Source: CAD feature listing. Evaluate the final solid. Frame: model axes, mm. Face numbers are marked on the shaded views. A direction names the side the tool comes from. Coordinates: 2 decimals unless noted, no trailing zeros. Order: outer loops, then holes, each group sorted by start corner. A loop starts at its lowest first (then second) coordinate and runs counter-clockwise, first axis right, second up. Notation, with made-up numbers: (21, 27) - (39, 27) arc R14 ccw to (39, 41) - close; hole circle Ø4 at (78, -23.5). An arc over 180 degrees is marked (long way). One line per question, with ' | ' between items. Start each with the question number.
(1) Contact query for flat-ended pins moving along their axis: P1, Ø1, axis at x = -7, y = 3, coming from the -Z side; P2, Ø0.6, axis at x = 0, z = 2, coming from the +Y side; P3, Ø1.6, axis at y = -9, z = 1.5, coming from the -X side. Output: stop coordinate, or through.
(2) Draft query along Y for the marked faces 1, 2 and 3. Return one class per face: +Y half, -Y half, draft (parallel to the pull), parting line (faces both ways), or undercut.
(3) Section B-B (x = 0). Return the cut outline in (y, z), then the cut area to 3 significant figures.
(4) Section A-A (z = 1.55). Return the cut outline in (x, y).
(5) Line query: line 1 along Y through (x, z) = (1.25, 1.35); line 2 along X through (y, z) = (5.75, 2); line 3 along X through (y, z) = (1.25, 2.65). Output: solid intervals per line, ascending.
(6) Access query for the marked faces 4, 5, 6 and 7. Directions: +Z, -Z, +X, -X, +Y, -Y. A direction counts if a zero-diameter tool reaches every point of the face in a straight line with its end or side. Return the directions, or none.
(7) Section D-D (y = 10). Return the cut outline in (x, z), then the cut area to 3 significant figures.
(8) Section C-C (y = 0). Return the cut outline in (x, z), then the cut area to 3 significant figures.
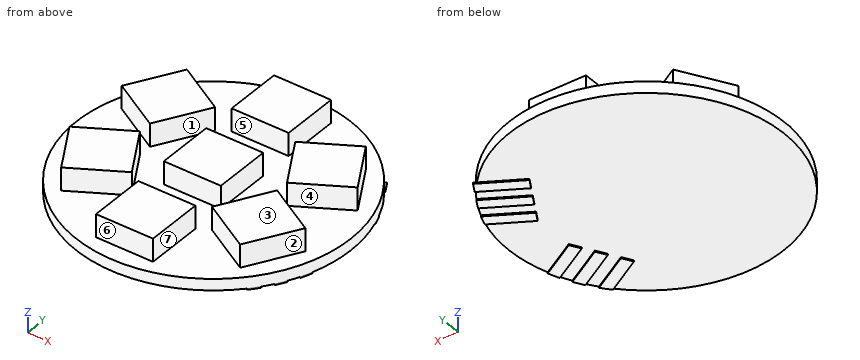
from build123d import *

# Parameters (mm, degrees)
CROQUIS1_R              = 12
SALIENTE_EXTRUIR1_DEPTH = 1
CROQUIS2_W              = 5
CROQUIS2_H              = 5
SALIENTE_EXTRUIR2_DEPTH = 2
SALIENTE_EXTRUIR3_DEPTH = 0.1


with BuildPart() as part:
    # Croquis1 → Saliente-Extruir1 (new body)
    with BuildSketch(Plane.XY):
        Circle(CROQUIS1_R)
    extrude(amount=SALIENTE_EXTRUIR1_DEPTH)

    # Croquis2 → Saliente-Extruir2 (add)
    with BuildSketch(Plane.XY.offset(1)):
        Rectangle(CROQUIS2_W, CROQUIS2_H)
        with Locations((0, -8)):
            Rectangle(CROQUIS2_W, CROQUIS2_H)
        with Locations((0, 8)):
            Rectangle(CROQUIS2_W, CROQUIS2_H)
        Polygon((-7.84326674, 7.415063509), (-10.34326674, 3.084936491), (-6.013139721, 0.584936491), (-3.513139721, 4.915063509), align=None)
        Polygon((-6.013139721, -0.584936491), (-10.34326674, -3.084936491), (-7.84326674, -7.415063509), (-3.513139721, -4.915063509), align=None)
        Polygon((6.013139721, -0.584936491), (3.513139721, -4.915063509), (7.84326674, -7.415063509), (10.34326674, -3.084936491), align=None)
        Polygon((7.84326674, 7.415063509), (3.513139721, 4.915063509), (6.013139721, 0.584936491), (10.34326674, 3.084936491), align=None)
    extrude(amount=SALIENTE_EXTRUIR2_DEPTH)

    # Croquis3 → Saliente-Extruir3 (add)
    with BuildSketch(Plane(origin=(0, 0, 0), x_dir=(-1, 0, 0), z_dir=(0, 0, -1))):
        with BuildLine():
            ThreePointArc((-9.560795314, -7.251978556), (-9.245794779, -7.649528018), (-8.914275675, -8.033410807))
            Line((-8.914275675, -8.033410807), (-5.67820323, -6.165063509))
            Line((-5.67820323, -6.165063509), (-6.17820323, -5.299038106))
            Line((-6.17820323, -5.299038106), (-9.560795314, -7.251978556))
        make_face()
        with BuildLine():
            Line((-7.17820323, -3.566987298), (-10.633279829, -5.561776702))
            ThreePointArc((-10.633279829, -5.561776702), (-10.515075861, -5.78214317), (-10.392305608, -5.999998679))
            ThreePointArc((-10.392305608, -5.999998679), (-10.265021594, -6.215249929), (-10.133279829, -6.427802106))
            Line((-10.133279829, -6.427802106), (-6.67820323, -4.433012702))
            Line((-6.67820323, -4.433012702), (-7.17820323, -3.566987298))
        make_face()
        with BuildLine():
            Line((-8.17820323, -1.834936491), (-11.414275675, -3.703283788))
            ThreePointArc((-11.414275675, -3.703283788), (-11.24758298, -4.182329148), (-11.060795314, -4.653902344))
            Line((-11.060795314, -4.653902344), (-7.67820323, -2.700961894))
            Line((-7.67820323, -2.700961894), (-8.17820323, -1.834936491))
        make_face()
        with BuildLine():
            Line((-7.67820323, 2.700961894), (-11.060795314, 4.653902344))
            ThreePointArc((-11.060795314, 4.653902344), (-11.24758298, 4.182329148), (-11.414275675, 3.703283788))
            Line((-11.414275675, 3.703283788), (-8.17820323, 1.834936491))
            Line((-8.17820323, 1.834936491), (-7.67820323, 2.700961894))
        make_face()
        with BuildLine():
            ThreePointArc((-10.133279829, 6.427802106), (-10.265021594, 6.215249929), (-10.392305608, 5.999998679))
            ThreePointArc((-10.392305608, 5.999998679), (-10.515075861, 5.78214317), (-10.633279829, 5.561776702))
            Line((-10.633279829, 5.561776702), (-7.17820323, 3.566987298))
            Line((-7.17820323, 3.566987298), (-6.67820323, 4.433012702))
            Line((-6.67820323, 4.433012702), (-10.133279829, 6.427802106))
        make_face()
        Polygon((-9.642304845, 7.299038106), (-6.17820323, 5.299038106), (-5.67820323, 6.165063509), (-9.142304845, 8.165063509), align=None)
    extrude(amount=SALIENTE_EXTRUIR3_DEPTH)


solid = part.part
Response values:
1) P1: stops at z = 0 | P2: stops at y = 10.5 | P3: stops at x = -8.59
2) face 1: undercut | face 2: -Y half | face 3: draft
3) outline: (-12, 0) - (12, 0) - (12, 1) - (10.5, 1) - (10.5, 3) - (5.5, 3) - (5.5, 1) - (2.5, 1) - (2.5, 3) - (-2.5, 3) - (-2.5, 1) - (-5.5, 1) - (-5.5, 3) - (-10.5, 3) - (-10.5, 1) - (-12, 1) - close | area: 54.0 mm²
4) outline: (-10.34, -3.08) - (-7.84, -7.42) - (-3.51, -4.92) - (-6.01, -0.58) - close; (-10.34, 3.08) - (-6.01, 0.58) - (-3.51, 4.92) - (-7.84, 7.42) - close; (-2.5, -10.5) - (2.5, -10.5) - (2.5, -5.5) - (-2.5, -5.5) - close; (-2.5, -2.5) - (2.5, -2.5) - (2.5, 2.5) - (-2.5, 2.5) - close; (-2.5, 5.5) - (2.5, 5.5) - (2.5, 10.5) - (-2.5, 10.5) - close; (3.51, -4.92) - (7.84, -7.42) - (10.34, -3.08) - (6.01, -0.58) - close; (3.51, 4.92) - (6.01, 0.58) - (10.34, 3.08) - (7.84, 7.42) - close
5) line 1: y = -10.5 to -5.5, -2.5 to 2.5, 5.5 to 10.5 | line 2: x = -8.8 to -4.96, -2.5 to 2.5, 4.96 to 8.8 | line 3: x = -7.17 to -5.63, -2.5 to 2.5, 5.63 to 7.17
6) face 4: +Z, +X | face 5: +Z | face 6: +Z, +X, -X, -Y | face 7: +Z, +Y, -Y
7) outline: (-6.63, 0) - (6.63, 0) - (6.63, 1) - (2.5, 1) - (2.5, 3) - (-2.5, 3) - (-2.5, 1) - (-6.63, 1) - close | area: 23.3 mm²
8) outline: (-12, 0) - (12, 0) - (12, 1) - (2.5, 1) - (2.5, 3) - (-2.5, 3) - (-2.5, 1) - (-12, 1) - close | area: 34.0 mm²
